Here's how the part is built. I have some questions about the finished solid (model axes, mm). Face numbers are marked on the shaded views. A direction names the side the tool comes from. Coordinates: 2 decimals unless noted, no trailing zeros. Write each loop counter-clockwise with the first axis right and the second up, starting at its lowest first coordinate (ties: lowest second). Pieces come first, ordered by that corner, then holes.
(1) Thinking about a two-plate mould opening in X: for the marked faces 3, 4 and 5, which applies, released by +X, released by -X, zero draft, split by the parting line, or undercut?
(2) Imagine slicing it at B-B, the plane y = -10. List the corners of the cut face in (x, z) for me.
(3) Imagine slicing it at D-D, the plane x = -4. List the corners of the cut face in (y, z) for me, plus the area to 3 significant figures.
(4) Imagine slicing it at C-C, the plane y = -4.75. List the corners of the cut face in (x, z) for me, plus the area to 3 significant figures.
(5) Please list where these lines run through material, in increasing order: probe 1 along X at (y, z) = (-20.75, 2.75); probe 2 along Y at (x, z) = (-0.5, 0); probe 3 along Z at (x, y) = (3.5, -8.25).
(6) For pin 1 Ø6 at (x, z) = (2.5, 4.5) entering from +Y; pin 2 Ø9.5 at (y, z) = (-10, 0) entering from +X; pin 3 Ø3 at (x, z) = (-3, -4.5) entering from +Y; pin 4 Ø6 at (x, z) = (-5, 6.5) entering from -Y, each with a flat end and sliding along its axis, tell me the tip position at first contact or that it passes through.
(7) Imagine slicing it at A-A, the plane z = 0. List the corners of the cut face in (x, y) for me, plus the area to 3 significant figures.
(8) Which directions (+Z, -Z, +X, -X, +Y, -Y) give clear straight access to the entire face, cutting with the end or side of a thin tool? Please do the marked faces 1 and 2.
```python
from build123d import *

# Parameters (mm, degrees)
SKETCH2_R          = 3
CUT_EXTRUDE1_DEPTH = 30.017236257


with BuildPart() as part:
    # Sketch1 → Revolve1 (revolve)
    with BuildSketch(Plane.XY, mode=Mode.PRIVATE) as revolve1_sk:
        Polygon((-6, 3), (-5, 3), (-5, 0), (5, 0), (5, 3), (6, 3), (6, -10), (-6, -10), align=None)
    revolve(revolve1_sk.sketch.rotate(Axis((-6, -10, 0), (1, 0, 0)), 90), axis=Axis((-6, -10, 0), (1, 0, 0)))

    # Sketch2 → Cut-Extrude1 (cut, through all)
    with BuildSketch(Plane.ZY.offset(6)):
        with Locations((0, -10)):
            Circle(SKETCH2_R)
    extrude(amount=-CUT_EXTRUDE1_DEPTH, mode=Mode.SUBTRACT)


solid = part.part
```
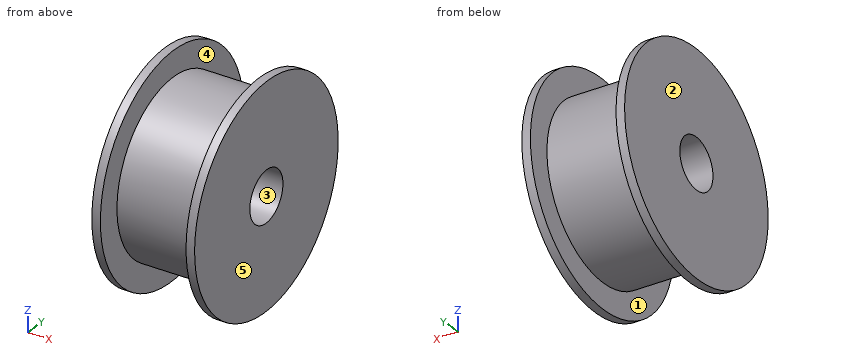
Recorded:
1. face 3: zero draft
1. face 4: undercut
1. face 5: released by +X
2. outline: (-6, -13) - (-5, -13) - (-5, -10) - (5, -10) - (5, -13) - (6, -13) - (6, -3) - (-6, -3) - close; (-6, 3) - (6, 3) - (6, 13) - (5, 13) - (5, 10) - (-5, 10) - (-5, 13) - (-6, 13) - close
3. outline: circle Ø20 at (-10, 0); hole circle Ø6 at (-10, 0)
3. area: 286 mm2
4. outline: (-6, -11.89) - (-5, -11.89) - (-5, -8.51) - (5, -8.51) - (5, -11.89) - (6, -11.89) - (6, 11.89) - (5, 11.89) - (5, 8.51) - (-5, 8.51) - (-5, 11.89) - (-6, 11.89) - close
4. area: 218 mm2
5. probe 1: x = -6 to -5, 5 to 6
5. probe 2: y = -20 to -13, -7 to 0
5. probe 3: z = -9.85 to -2.44, 2.44 to 9.85
6. pin 1: stops at y = 2.69
6. pin 2: stops at x = 6
6. pin 3: stops at y = -0.46
6. pin 4: stops at y = -22.52
7. outline: (-6, -23) - (-5, -23) - (-5, -20) - (5, -20) - (5, -23) - (6, -23) - (6, -13) - (-6, -13) - close; (-6, -7) - (6, -7) - (6, 3) - (5, 3) - (5, 0) - (-5, 0) - (-5, 3) - (-6, 3) - close
7. area: 180 mm2
8. face 1: none
8. face 2: +Z, -Z, -X, +Y, -Y
